The listing builds one solid part. Answer for the finished solid, in the listing's coordinates (mm). A direction names the side the tool comes from. Coordinates: 2 decimals unless noted, no trailing zeros. Write each loop counter-clockwise with the first axis right and the second up, starting at its lowest first coordinate (ties: lowest second). Pieces come first, ordered by that corner, then holes.
from build123d import *

# Parameters (mm, degrees)
SKETCH_W        = 125
SKETCH_H        = 115
PAD_DEPTH       = 4
SKETCH001_W     = 121
SKETCH001_H     = 111
POCKET_DEPTH    = 2.3
SKETCH002_W     = 74
SKETCH002_H     = 44
PAD001_DEPTH    = 13
CHAMFER_SIZE    = 2
SKETCH003_W     = 70
SKETCH003_H     = 40
POCKET001_DEPTH = 11
SKETCH004_W     = 49.7
SKETCH004_H     = 38
PAD002_DEPTH    = 5
POCKET002_DEPTH = 76.501
SKETCH006_W     = 49.9508758682
SKETCH006_H     = 38
SKETCH006_R     = 2
SKETCH006_W_2   = 35
SKETCH006_H_2   = 35
PAD003_DEPTH    = 7
SKETCH007_W     = 35
SKETCH007_H     = 35
POCKET003_DEPTH = 25.6742234963


with BuildPart() as part:
    # Sketch → Pad (new body)
    with BuildSketch(Plane.XY):
        with Locations((62.5, 57.5)):
            Rectangle(SKETCH_W, SKETCH_H)
    extrude(amount=PAD_DEPTH)

    # Sketch001 (on Face6 of Pad) → Pocket (cut)
    with BuildSketch(Plane.XY.offset(4)):
        with Locations((62.5, 57.5)):
            Rectangle(SKETCH001_W, SKETCH001_H)
    extrude(amount=-POCKET_DEPTH, mode=Mode.SUBTRACT)

    # Sketch002 (on Face4 of Pocket) → Pad001 (join)
    with BuildSketch(Plane(origin=(0, 0, 0), x_dir=(1, 0, 0), z_dir=(0, 0, -1))):
        with Locations((62.5, -57.5)):
            Rectangle(SKETCH002_W, SKETCH002_H)
    extrude(amount=PAD001_DEPTH)

    # Chamfer
    chamfer_edges = [part.edges().sort_by_distance(p)[0] for p in [
        (62.5, 35.5, 0),
        (99.5, 57.5, 0),
        (62.5, 79.5, 0),
        (25.5, 57.5, 0),
    ]]
    chamfer(chamfer_edges, length=CHAMFER_SIZE)

    # Sketch003 (on Face20 of Chamfer) → Pocket001 (cut)
    with BuildSketch(Plane.XY.offset(1.7)):
        with Locations((62.5, 57.5)):
            Rectangle(SKETCH003_W, SKETCH003_H)
    extrude(amount=-POCKET001_DEPTH, mode=Mode.SUBTRACT)

    # Sketch004 (on Face15 of Pocket001) → Pad002 (join)
    with BuildSketch(Plane(origin=(0, 0, -13), x_dir=(1, 0, 0), z_dir=(0, 0, -1))):
        with Locations((62.35, -57.5)):
            Rectangle(SKETCH004_W, SKETCH004_H)
    extrude(amount=PAD002_DEPTH)

    # Sketch005 (on Face22 of Pad002) → Pocket002 (cut, through all)
    with BuildSketch(Plane(origin=(0, 76.5, 0), x_dir=(-1, 0, 0), z_dir=(0, 1, 0))):
        Polygon((-37.5, -13), (-87.2, -18), (-37.5, -18), align=None)
    extrude(amount=-POCKET002_DEPTH, mode=Mode.SUBTRACT)

    # Sketch006 (on Face23 of Pocket002) → Pad003 (join)
    with BuildSketch(Plane(origin=(-0.9190049257, 0, -9.1349089612), x_dir=(0.9949775482, 0, -0.1000983449), z_dir=(-0.1000983449, 0, -0.9949775482))):
        with Locations((63.5883744738, -57.5)):
            Rectangle(SKETCH006_W, SKETCH006_H)
        with Locations((42.3629365397, -47.5)):
            Circle(SKETCH006_R, mode=Mode.SUBTRACT)
        with Locations((42.3629365397, -67.5)):
            Circle(SKETCH006_R, mode=Mode.SUBTRACT)
        with Locations((84.8629365397, -47.5)):
            Circle(SKETCH006_R, mode=Mode.SUBTRACT)
        with Locations((84.8629365397, -67.5)):
            Circle(SKETCH006_R, mode=Mode.SUBTRACT)
        with Locations((63.6129365397, -57.5)):
            Rectangle(SKETCH006_W_2, SKETCH006_H_2, mode=Mode.SUBTRACT)
    extrude(amount=PAD003_DEPTH)

    # Sketch007 (on Face38 of Pad003) → Pocket003 (cut, through all)
    with BuildSketch(Plane(origin=(-0.9190049257, 0, -9.1349089612), x_dir=(0.9949775482, 0, -0.1000983449), z_dir=(-0.1000983449, 0, -0.9949775482))):
        with Locations((63.6129365397, -57.5)):
            Rectangle(SKETCH007_W, SKETCH007_H)
    extrude(amount=-POCKET003_DEPTH, mode=Mode.SUBTRACT)


solid = part.part
1. Section C-C on y = 43 is taken. Give the vertices of the cut face in (x, z), then the cut area to 3 significant figures.
Results found:
outline: (0, 0) - (23.5, 0) - (25.5, -2) - (25.5, -13) - (37.5, -13) - (36.8, -19.96) - (44.26, -20.72) - (45.41, -9.3) - (27.5, -9.3) - (27.5, 1.7) - (2, 1.7) - (2, 4) - (0, 4) - close; (79.09, -24.22) - (86.5, -24.96) - (87.2, -18) - (87.2, -13) - (99.5, -13) - (99.5, -2) - (101.5, 0) - (125, 0) - (125, 4) - (123, 4) - (123, 1.7) - (97.5, 1.7) - (97.5, -9.3) - (80.59, -9.3) - close
area: 428 mm2
2. Section D-D on x = 71.5 is taken. Give the vertices of the cut face in (y, z), then the cut area to 3 significant figures.
Results found:
outline: (0, 0) - (33.5, 0) - (35.5, -2) - (35.5, -13) - (38.5, -13) - (38.5, -23.46) - (40, -23.46) - (40, -9.3) - (37.5, -9.3) - (37.5, 1.7) - (2, 1.7) - (2, 4) - (0, 4) - close; (75, -23.46) - (76.5, -23.46) - (76.5, -13) - (79.5, -13) - (79.5, -2) - (81.5, 0) - (115, 0) - (115, 4) - (113, 4) - (113, 1.7) - (77.5, 1.7) - (77.5, -9.3) - (75, -9.3) - close
area: 243 mm2
3. Flat-ended cylindrical pins translate along their axes: P1, Ø3.5, axis at y = 53.5, z = -6, coming from the -X side; P2, Ø4.5, axis at x = 59.5, z = -16.5, coming from the -Y side; P3, Ø5.5, axis at y = 68, z = -6, coming from the +X side. Find the tip coordinate at first contact, or state that the pin passes through.
Results found:
P1: stops at x = 25.5
P2: stops at y = 38.5
P3: stops at x = 99.5
4. Section B-B on y = 87 is taken. Give the vertices of the cut face in (x, z).
Results found:
outline: (0, 0) - (125, 0) - (125, 4) - (123, 4) - (123, 1.7) - (2, 1.7) - (2, 4) - (0, 4) - close
5. Section A-A on z = -4.5 is taken. Give the vertices of the cut face in (x, y).
Results found:
outline: (25.5, 35.5) - (99.5, 35.5) - (99.5, 79.5) - (25.5, 79.5) - close; hole (27.5, 37.5) - (97.5, 37.5) - (97.5, 77.5) - (27.5, 77.5) - close
6. Find the intervals of material crossed by L1, parallel to Y at x = 66.5, z = -19.75; L2, parallel to Y at x = 53.5, z = 1; L3, parallel to X at y = 77, z = -9.25, in increasing order.
Results found:
L1: y = 38.5 to 40, 75 to 76.5
L2: y = 0 to 37.5, 77.5 to 115
L3: x = 25.5 to 27.5, 97.5 to 99.5
7. A tool of negligible diameter and unlimited length cuts with its end or side. For faces 5 (the flat face through (62, 83, 1.7)), 6 (the flat face through (83.49, 47.528, -17.627)), 7 (the flat face through (99.5, 58, -7)), from which of +Z, -Z, +X, -X, +Y, -Y can it reach the whole face along a straight path? Write none if from no direction.
Results found:
face 5: +Z
face 6: none
face 7: -Z, +X, +Y, -Y
8. For a pull along Z with two mould halves and no side action, classify faces 1 (the flat face through (62, 38.5, -18)), 2 (the flat face through (57.852, 75.708, -22.083)), 3 (the flat face through (62, 76, -9.3)), 4 (the flat face through (37.155, 57.766, -16.434)) as pulls with the +Z half, pulls with the -Z half, needs draft (parallel to the pull), parting line crosses it, or undercut.
Results found:
face 1: needs draft
face 2: pulls with the -Z half
face 3: pulls with the +Z half
face 4: undercut
